Can you work these out from the model? Positions are in its coordinate system, mm. A direction names the side the tool comes from. Round coordinates to 2 decimals unless told otherwise and drop trailing zeros. Order: outer loops, then holes, each group sorted by start corner. A loop starts at its lowest first (then second) coordinate and runs counter-clockwise, first axis right, second up. Notation, with made-up numbers: (47, 45.25) - (70, 45.25) arc R22 ccw to (70, 77.25) - close; hole circle Ø9 at (8.5, 38.25). An arc over 180 degrees is marked (long way). Write item = value, one per line.
from build123d import *

# Parameters (mm, degrees)
F0_W     = 3.9895381778
F0_H     = 12.3155266047
F0_W_2   = 3.8160792319
F0_H_2   = 13.7031897902
F0_W_3   = 24.9779764563
F0_H_3   = 5.550660193
F0_W_4   = 26.0187210515
F0_H_4   = 5.897577852
F0_H_5   = 3.1222477555
F0_H_6   = 2.2549591959
F0_W_5   = 2.2549559362
F0_W_6   = 3.8160814438
F0_W_7   = 18.7334809452
F0_H_7   = 12.6624442637
F0_W_8   = 20.6415196881
F0_H_8   = 12.1420696378
F1_DEPTH = 3


with BuildPart() as f1:
    # F0 (on Front) → F1 (new body)
    with BuildSketch(Plane.XZ):
        with Locations((-5.6373900734, -65.0468096137)):
            Rectangle(F0_W, F0_H)
        with Locations((3.1222468824, -65.7406412065)):
            Rectangle(F0_W_2, F0_H_2)
        with Locations((-21.508811973, -46.5735159814)):
            Rectangle(F0_W_3, F0_H_3)
        with Locations((19.7742297314, -46.4000571519)):
            Rectangle(F0_W_4, F0_H_4)
        Polygon((-9.0198237449, -34.7783602774), (-9.0198237449, -38.0706993256), (6.7648692057, -37.4577013494), (6.7648692057, -34.7783602774), align=None)
        with Locations((-5.6373900734, -57.3279224336)):
            Rectangle(F0_W, F0_H_5)
        with Locations((3.1222468824, -57.7615667135)):
            Rectangle(F0_W_2, F0_H_6)
        with Locations((-7.8923457768, -46.5735159814)):
            Rectangle(F0_W_5, F0_H_3)
        with Locations((4.8568284838, -46.4000571519)):
            Rectangle(F0_W_6, F0_H_4)
        Polygon((6.7648692057, -37.4577013494), (-9.0198237449, -38.0706993256), (-9.0198237449, -43.798185885), (-6.7648678087, -43.798185885), (-6.7648678087, -49.3488460779), (-9.0198237449, -49.3488460779), (-9.0198237449, -58.8890463114), (-7.6321591623, -58.8890463114), (-7.6321591623, -55.7667985559), (-3.6426209845, -55.7667985559), (-3.6426209845, -58.8890463114), (1.2142072665, -58.8890463114), (1.2142072665, -56.6340871155), (5.0302864984, -56.6340871155), (5.0302864984, -58.8890463114), (6.7648692057, -58.8890463114), (6.7648692057, -49.3488460779), (2.9487877619, -49.3488460779), (2.9487877619, -43.4512682259), (6.7648692057, -43.4512682259), align=None)
        Polygon((-55.3331524134, 46.7469729483), (-55.3331524134, -39.8086495697), (-53.7720285356, -39.8086495697), (-9.0198237449, -38.0706993256), (-9.0198237449, -34.7783602774), (6.7648692057, -34.7783602774), (6.7648692057, -37.4577013494), (53.4251108766, -35.6456525624), (53.4251108766, 46.7469729483), align=None)
        with Locations((-29.6613452956, 31.742842868)):
            Rectangle(F0_W_7, F0_H_7, mode=Mode.SUBTRACT)
        Polygon((-5.2037448622, 30.4419063032), (-19.6007713675, 43.1043542922), (-14.2235690728, 43.4512682259), (-3.0722282925, 36.8575679841), (6.0710357502, 43.4512682259), (12.8359030932, 43.4512682259), align=None, mode=Mode.SUBTRACT)
        Polygon((-33.824339509, -16.2183362991), (-33.824339509, 8.2392627373), (-18.7334809452, 8.2392627373), (-18.7334809452, -12.5757167116), (21.5088110417, -12.5757167116), (21.5088110417, 8.9330952615), (34.1712571681, 8.9330952615), (34.1712571681, -17.6060032099), (26.192182675, -17.6060032099), (26.192182675, -25.7585346699), (-28.6205969751, -25.7585346699), (-28.6205969751, -16.2183362991), align=None, mode=Mode.SUBTRACT)
        with Locations((23.850497324, 33.2172363997)):
            Rectangle(F0_W_8, F0_H_8, mode=Mode.SUBTRACT)
    extrude(amount=F1_DEPTH)


solid = f1.part
(1) On a 3-axis mill with a long thin cutter (end or side, diameter ignored), from which of +Z, -Z, +X, -X, +Y, -Y can I reach the whole of each face in a straight line? I mean faces 1 (the face through (6.765, -1, -54)), 2 (the face through (-9.02, -1, -54)), 3 (the face through (1.214, -1, -66)), 4 (the face through (-39.028, -1, 32)). Say none if no direction works.
Computed:
face_1 = -Z, +X, +Y, -Y
face_2 = -Z, -X, +Y, -Y
face_3 = -Z, +Y, -Y
face_4 = +Y, -Y
(2) If we section it at C-C (y = -1.2): State how many separate pieces and enclosed holes the cut face has, plus the area to 3 significant figures.
Computed:
separate_pieces = 1
enclosed_holes = 4
area = 7,920 mm^2
(3) If we section it at A-A (x = -30): Write out the boundary of the cut face in (y, z), plus the area to 3 significant figures.
Computed:
outline = (-3, -49.35) - (0, -49.35) - (0, -43.8) - (-3, -43.8) - close; (-3, -38.89) - (0, -38.89) - (0, -16.22) - (-3, -16.22) - close; (-3, 8.24) - (0, 8.24) - (0, 25.41) - (-3, 25.41) - close; (-3, 38.07) - (0, 38.07) - (0, 46.75) - (-3, 46.75) - close
area = 162 mm^2
(4) Will these pins go through, and if not, where does the flat tip stop? P1, Ø0.9, axis at x = 25.5, y = -1.5, coming from the -Z side; P2, Ø1.5, axis at y = -1.5, z = -46.5, coming from the +X side.
Computed:
P1 = -49.35
P2 = 32.78
(5) Thinking about a two-plate mould opening in Z: for faces 5 (the face through (20, -1, -43.451)), 6 (the face through (-1, -1, -58.889)), 7 (the face through (-21, -1, -43.798)), 8 (the face through (5.03, -1, -66)), which applies, +Z half, -Z half, draft (parallel to the pull), parting line (faces both ways), or undercut?
Computed:
face_5 = undercut
face_6 = -Z half
face_7 = undercut
face_8 = draft
(6) If we section it at B-B (x = 3): Write out the boundary of the cut face in (y, z), plus the area to 3 significant figures.
Computed:
outline = (-3, -72.59) - (0, -72.59) - (0, -25.76) - (-3, -25.76) - close; (-3, -12.58) - (0, -12.58) - (0, 36.36) - (-3, 36.36) - close; (-3, 41.24) - (0, 41.24) - (0, 46.75) - (-3, 46.75) - close
area = 304 mm^2
(7) If we section it at D-D (z = 34.5): Write out the boundary of the cut face in (x, y), plus the area to 3 significant figures.
Computed:
outline = (-55.33, -3) - (-39.03, -3) - (-39.03, 0) - (-55.33, 0) - close; (-20.29, -3) - (-9.82, -3) - (-9.82, 0) - (-20.29, 0) - close; (0.42, -3) - (13.53, -3) - (13.53, 0) - (0.42, 0) - close; (34.17, -3) - (53.43, -3) - (53.43, 0) - (34.17, 0) - close
area = 177 mm^2
(8) If I drill on line 1 (X direction, y = -2.6, z = -3); line 2 (X direction, y = -2.4, z = -68); line 3 (Z direction, x = 22, y = -2.3), over which ranges is the centre line in solid material (lowest first)? Write a range as from..to.
Computed:
line_1 = -55.33..-33.82, -18.73..21.51, 34.17..53.43
line_2 = -7.63..-3.64, 1.21..5.03
line_3 = -49.35..-43.45, -36.87..-25.76, 8.93..27.15, 39.29..46.75
